Verification items for this drawing (mm, ordinates from the low corner). A direction names the side the tool comes from. Round coordinates to 2 decimals unless told otherwise and drop trailing zeros. Loops run counter-clockwise (first coordinate to the right, second up) from the corner with the lowest first, then second, coordinate; pieces in that order, holes last. Notation, with made-up numbers: M -37,61 L 15,61 A11 cw 15,75 Z; hole C 72,7 d6. An arc over 180 degrees is marked long. Answer in a Markdown table with one row per item. Add a question column.
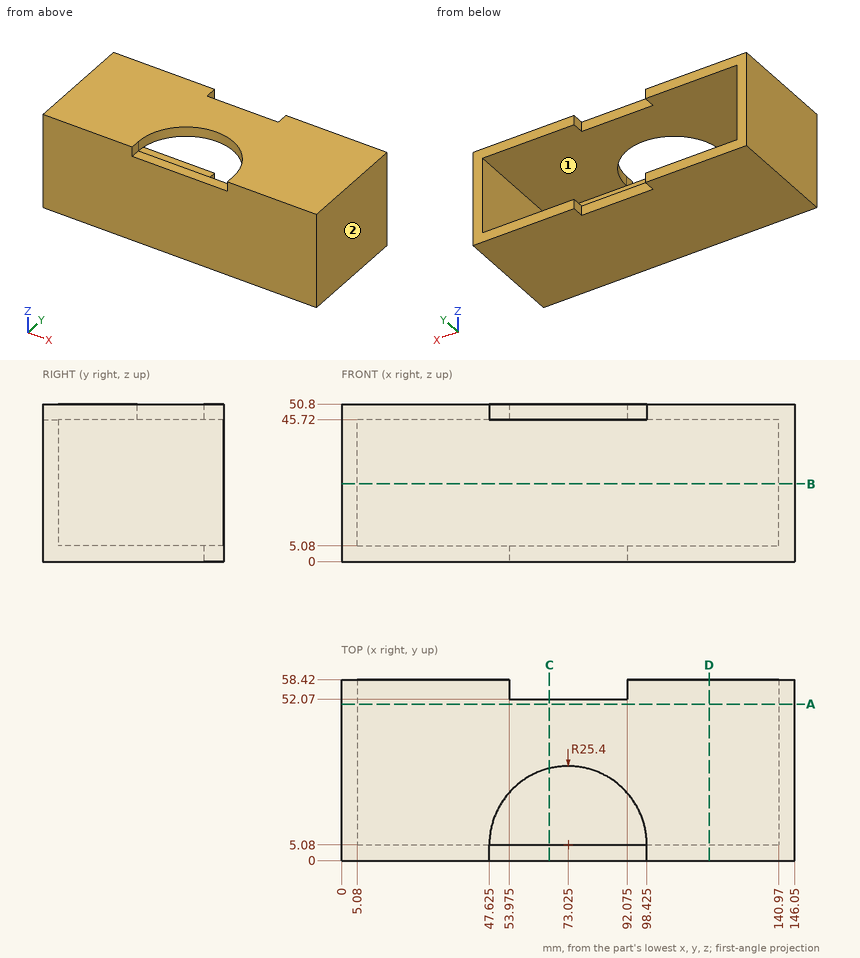
1) Cross-section at B-B, the plane z = 25. Record the boundary of the cut face in (x, y).
2) Go/stop test with flat-tipped pins: pin 1 (2.5 mm diameter, centred on x = 80, z = 47, fed in from +Y); pin 2 (3 mm diameter, centred on x = 114.5, y = 31.5, fed in from -Z); pin 3 (12 mm diameter, centred on x = 87.5, z = 26, fed in from +Y); pin 4 (1.5 mm diameter, centred on x = 82.5, y = 1.5, fed in from +Z). Record where each tip stops, or that it passes through.
3) Cross-section at D-D, the plane x = 118.5. Record the boundary of the cut face in (y, z), plus the area to 3 significant figures.
4) Set-up check for the marked faces 1 and 2: record each of +Z, -Z, +X, -X, +Y, -Y from which the full face is reachable in a straight line by a thin tool's end or side.
5) Cross-section at A-A, the plane y = 50.5. Record the boundary of the cut face in (x, z), plus the area to 3 significant figures.
6) Cross-section at C-C, the plane x = 67. Record the boundary of the cut face in (y, z), plus the area to 3 significant figures.
7) Thickness scan on L1, parallel to X at y = 50.5, z = 36.5; L2, parallel to Z at x = 35.5, y = 55; L3, parallel to Y at x = 94, z = 14. Record the ranges inside material, lowest first. Write a range as [from, to].
Worked answers:
| question | item | result |
|---|---|---|
| 1 | outline | M 0,0 L 146.05,0 L 146.05,58.42 L 140.97,58.42 L 140.97,5.08 L 5.08,5.08 L 5.08,58.42 L 0,58.42 Z |
| 2 | pin 1 | stops at y = 52.07 |
| 2 | pin 2 | stops at z = 0 |
| 2 | pin 3 | stops at y = 5.08 |
| 2 | pin 4 | stops at z = 45.72 |
| 3 | outline | M 0,0 L 58.42,0 L 58.42,5.08 L 5.08,5.08 L 5.08,45.72 L 58.42,45.72 L 58.42,50.8 L 0,50.8 Z |
| 3 | area | 800 mm2 |
| 4 | face 1 | +Y |
| 4 | face 2 | +Z, -Z, +X, +Y, -Y |
| 5 | outline | M 0,0 L 146.05,0 L 146.05,50.8 L 0,50.8 Z; hole M 5.08,5.08 L 140.97,5.08 L 140.97,45.72 L 5.08,45.72 Z |
| 5 | area | 1,900 mm2 |
| 6 | outline | M 0,0 L 52.07,0 L 52.07,5.08 L 5.08,5.08 L 5.08,45.72 L 0,45.72 Z; M 29.76,45.72 L 52.07,45.72 L 52.07,50.8 L 29.76,50.8 Z |
| 6 | area | 584 mm2 |
| 7 | L1 | x = [0, 5.08], [140.97, 146.05] |
| 7 | L2 | z = [0, 5.08], [45.72, 50.8] |
| 7 | L3 | y = [0, 5.08] |
